from build123d import *

# Parameters (mm, degrees)
BOSS_EXTRUDE1_DEPTH = 3.5
BOSS_EXTRUDE2_DEPTH = 7
SKETCH6_W           = 34
SKETCH6_H           = 10
CUT_EXTRUDE1_DEPTH  = 7
SKETCH7_R           = 7
CUT_EXTRUDE2_DEPTH  = 7
CUT_EXTRUDE3_DEPTH  = 7
SKETCH11_W          = 113
SKETCH11_H          = 23.8
CUT_EXTRUDE4_DEPTH  = 7


with BuildPart() as part:
    # Sketch1 → Boss-Extrude1 (new body, symmetric)
    with BuildSketch(Plane(origin=(0, 0, 0), x_dir=(1, 0, 0), z_dir=(0, 1, 0))):
        Polygon((90, 0), (-90, 0), (-90, -70), (-25, -115), (-25, -165), (-66.5, -165), (-66.5, -195), (66.5, -195), (66.5, -165), (25, -165), (25, -115), (90, -70), align=None)
    extrude(amount=BOSS_EXTRUDE1_DEPTH, both=True)

    # Sketch2 → Boss-Extrude2 (add)
    with BuildSketch(Plane(origin=(0, 3.5, 0), x_dir=(1, 0, 0), z_dir=(0, 1, 0))):
        with BuildLine():
            Line((-66.5, -165), (-66.5, -195))
            ThreePointArc((-66.5, -195), (-83.296215978, -173.392103188), (-82.268838739, -146.043271918))
            ThreePointArc((-82.268838739, -146.043271918), (-76.884146381, -157.600992268), (-66.5, -165))
        make_face()
        with BuildLine():
            Line((66.5, -165), (66.5, -195))
            ThreePointArc((66.5, -195), (83.296215978, -173.392103188), (82.268838739, -146.043271918))
            ThreePointArc((82.268838739, -146.043271918), (76.884146381, -157.600992268), (66.5, -165))
        make_face()
    extrude(amount=-BOSS_EXTRUDE2_DEPTH)

    # Sketch6 → Cut-Extrude1 (cut)
    with BuildSketch(Plane(origin=(0, 3.5, 0), x_dir=(1, 0, 0), z_dir=(0, 1, 0))):
        with Locations((0, -160)):
            Rectangle(SKETCH6_W, SKETCH6_H)
        with Locations((0, -120)):
            Rectangle(SKETCH6_W, SKETCH6_H)
    extrude(amount=-CUT_EXTRUDE1_DEPTH, mode=Mode.SUBTRACT)

    # Sketch7 → Cut-Extrude2 (cut)
    with BuildSketch(Plane(origin=(0, 3.5, 0), x_dir=(1, 0, 0), z_dir=(0, 1, 0))):
        with Locations((0, -140)):
            Circle(SKETCH7_R)
    extrude(amount=-CUT_EXTRUDE2_DEPTH, mode=Mode.SUBTRACT)

    # Sketch9 → Cut-Extrude3 (cut)
    with BuildSketch(Plane(origin=(0, 3.5, 0), x_dir=(1, 0, 0), z_dir=(0, 1, 0))):
        Polygon((-34, -75), (-73.695942788, -75), (-34, -104.097660068), align=None)
        Polygon((34, -104.097660068), (34, -75), (73.695942788, -75), align=None)
    extrude(amount=-CUT_EXTRUDE3_DEPTH, mode=Mode.SUBTRACT)

    # Sketch11 → Cut-Extrude4 (cut)
    with BuildSketch(Plane(origin=(0, 3.5, 0), x_dir=(1, 0, 0), z_dir=(0, 1, 0))):
        with Locations((0, -183.1)):
            Rectangle(SKETCH11_W, SKETCH11_H)
    extrude(amount=-CUT_EXTRUDE4_DEPTH, mode=Mode.SUBTRACT)


solid = part.part
Can you work these out from the model? Positions are in its coordinate system, mm. A direction names the side the tool comes from. Give positions to 0.01 mm unless a question says otherwise; leave off trailing zeros. Order: outer loops, then holes, each group sorted by start corner. A loop starts at its lowest first (then second) coordinate and runs counter-clockwise, first axis right, second up. Notation, with made-up numbers: (69, 39) - (92, 39) arc R22 cw to (92, 77) - close; hole circle Ø11 at (-40, -2). An arc over 180 degrees is marked (long way). Write each question's results on one line, items separated by ' | '.
1) Please list where these lines run through material, in increasing order: line 1 along Z through (x, y) = (-12, 0); line 2 along Z through (x, y) = (0, -1.25); line 3 along X through (y, z) = (-1.25, 140). Write a range as [from, to].
Final values:
line 1: z = [0, 115], [125, 155], [165, 171.2] | line 2: z = [0, 115], [125, 133], [147, 155], [165, 171.2] | line 3: x = [-25, -7], [7, 25]
2) On a 3-axis mill with a long thin cutter (end or side, diameter ignored), from which of +Z, -Z, +X, -X, +Y, -Y can I reach the whole of each face in a straight line? I mean faces 1 (the face through (-56.5, 0, 183)), 2 (the face through (54, 0, 75)), 3 (the face through (-62, 0, 195)). Say none if no direction works.
Final values:
face 1: +Z, +Y, -Y | face 2: +Y, -Y | face 3: +Z, +X, -X, +Y, -Y
3) Suppose I cut it at A-A, the plane x = 0. Write out the boundary of the cut face in (y, z), then the cut area to 3 significant figures.
Final values:
outline: (-3.5, 0) - (3.5, 0) - (3.5, 115) - (-3.5, 115) - close; (-3.5, 125) - (3.5, 125) - (3.5, 133) - (-3.5, 133) - close; (-3.5, 147) - (3.5, 147) - (3.5, 155) - (-3.5, 155) - close; (-3.5, 165) - (3.5, 165) - (3.5, 171.2) - (-3.5, 171.2) - close | area: 960 mm^2
4) I'm going to push flat-ended pins straight in: pin 1 Ø3.5 at (y, z) = (0, 127.5) entering from -X; pin 2 Ø3 at (y, z) = (1.5, 166) entering from +X; pin 3 Ø3.5 at (x, y) = (14, 0) entering from +Z; pin 4 Ø2 at (x, y) = (-3, 0) entering from -Z. Where does each tip first touch, or does it pass through?
Final values:
pin 1: stops at x = -25 | pin 2: stops at x = 85.08 | pin 3: stops at z = 171.2 | pin 4: stops at z = 0
5) Suppose I cut it at B-B, the plane y = 0.5. Give the number of separate pieces and of enclosed holes in the cut face, then the cut area to 3 significant figures.
Final values:
separate pieces: 1 | enclosed holes: 5 | area: 20,600 mm^2
6) Suppose I cut it at D-D, the plane x = -61.5. Write out the boundary of the cut face in (y, z).
Final values:
outline: (-3.5, 0) - (3.5, 0) - (3.5, 75) - (-3.5, 75) - close; (-3.5, 83.94) - (3.5, 83.94) - (3.5, 89.73) - (-3.5, 89.73) - close; (-3.5, 165) - (3.5, 165) - (3.5, 195) - (-3.5, 195) - close
7) Suppose I cut it at C-C, the plane z = 140. Write out the boundary of the cut face in (x, y), then the cut area to 3 significant figures.
Final values:
outline: (-25, -3.5) - (-7, -3.5) - (-7, 3.5) - (-25, 3.5) - close; (7, -3.5) - (25, -3.5) - (25, 3.5) - (7, 3.5) - close | area: 252 mm^2
8) If we mould it in two halves opening along Z, with no side actions, what happens to faces 4 (the face through (77, 0.05, 157.46)), 5 (the face through (-90, 0, 35)), 6 (the face through (1, 0, 0))? For each: pulls with the +Z half, pulls with the -Z half, needs draft (parallel to the pull), parting line crosses it, or undercut.
Final values:
face 4: undercut | face 5: needs draft | face 6: pulls with the -Z half
